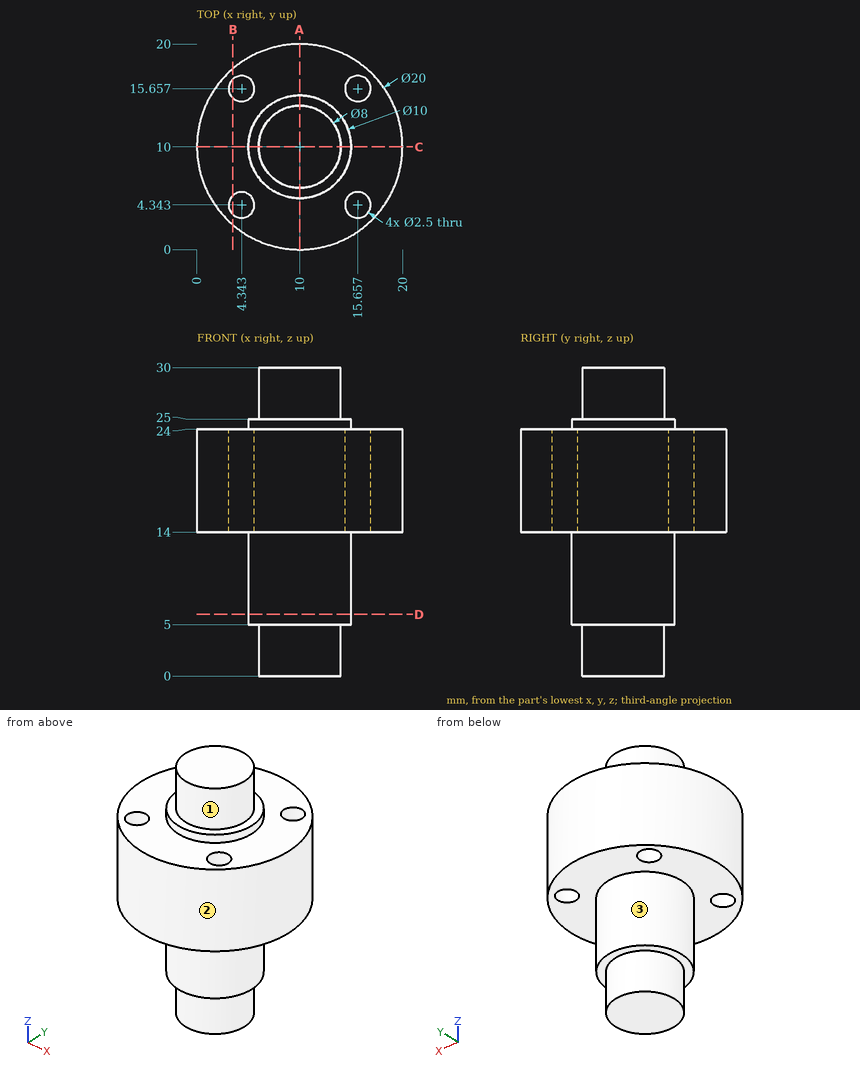
Check sheet for the drawn part. Datum: minimum x, y, z corner. Units: mm. A direction names the side the tool comes from. Give positions to 0.01 mm unless a question says otherwise; leave off trailing zeros. Write each loop counter-clockwise with the first axis right and the second up, starting at its lowest first coordinate (ties: lowest second). Pieces come first, ordered by that corner, then holes.
(1) Gauge pin test, flat ends, axial feed: pin 1 (2 mm diameter, centred on x = 15.66, y = 15.66, fed in from -Z); pin 2 (6 mm diameter, centred on y = 12.5, z = 26.5, fed in from +X); pin 3 (4 mm diameter, centred on x = 15.66, y = 4.34, fed in from -Z); pin 4 (1.5 mm diameter, centred on x = 2.5, z = 23, fed in from -Y). Record the tip position at first contact, or that the pin passes through.
(2) Cross-section at B-B (x = 3.5). Enter the section's corners in (y, z).
(3) Material ranges on line 1 (Y direction, x = 4.75, z = 22.5) (1 decimal); line 2 (Z direction, x = 5.5, y = 5.25); line 3 (Z direction, x = 9.5, y = 14.5), recorded low to high.
(4) Cross-section at A-A (x = 10). Enter the section's corners in (y, z), plus the area to 3 significant figures.
(5) Access from +Z, -Z, +X, -X, +Y, -Y to the whole of each face (thin tool, end or side, straight path). Record for the marked faces 1, 2 and 3.
(6) Cross-section at D-D (z = 6). Enter the section's corners in (x, y), plus the area to 3 significant figures.
Worked out:
1. pin 1: passes through
1. pin 2: stops at x = 19.96
1. pin 3: stops at z = 14
1. pin 4: stops at y = 2.62
2. outline: (2.4, 14) - (3.42, 14) - (3.42, 24) - (2.4, 24) - close; (5.27, 14) - (14.73, 14) - (14.73, 24) - (5.27, 24) - close; (16.58, 14) - (17.6, 14) - (17.6, 24) - (16.58, 24) - close
3. line 1: y = 1.5 to 3.2, 5.5 to 14.5, 16.8 to 18.5
3. line 2: z = 14 to 24
3. line 3: z = 5 to 25
4. outline: (0, 14) - (5, 14) - (5, 5) - (6, 5) - (6, 0) - (14, 0) - (14, 5) - (15, 5) - (15, 14) - (20, 14) - (20, 24) - (15, 24) - (15, 25) - (14, 25) - (14, 30) - (6, 30) - (6, 25) - (5, 25) - (5, 24) - (0, 24) - close
4. area: 380 mm2
5. face 1: +Z
5. face 2: +Z, -Z
5. face 3: -Z
6. outline: circle Ø10 at (10, 10)
6. area: 78.5 mm2
